Can you work these out from the drawing? Everything is in mm from the part's minimum corner. A direction names the side the tool comes from. Give positions to 0.01 mm unless a question says otherwise; leave off trailing zeros.
Q1. We'd pull the mould along X, two halves only. Please class the marked faces 3, 4 and 5: +X half, -X half, draft (parallel to the pull), parting line (faces both ways), or undercut.
Q2. For the marked faces 1 and 2, which set-ups out of +Z, -Z, +X, -X, +Y, -Y let a thin tool reach every point of the face, with its end or its side?
Q3. If we section it at A-A (y = 5): Give the number of separate pieces and of enclosed holes in the cut face.
Q4. I need wall thicknesses on line 1 (Z direction, x = 1.5, y = 5.75); line 2 (X direction, y = 6.25, z = 1.65); line 3 (Y direction, x = 14.75, z = 1.7) (1 decimal). Which ranges of each line are inside material? Lowest first, please.
Q5. Will these pins go through, and if not, where does the flat tip stop? P1, Ø2, axis at x = 12, z = 1, coming from the +Y side (1 decimal); P2, Ø1.5, axis at x = 6.5, z = 1, coming from the -Y side (1 decimal).
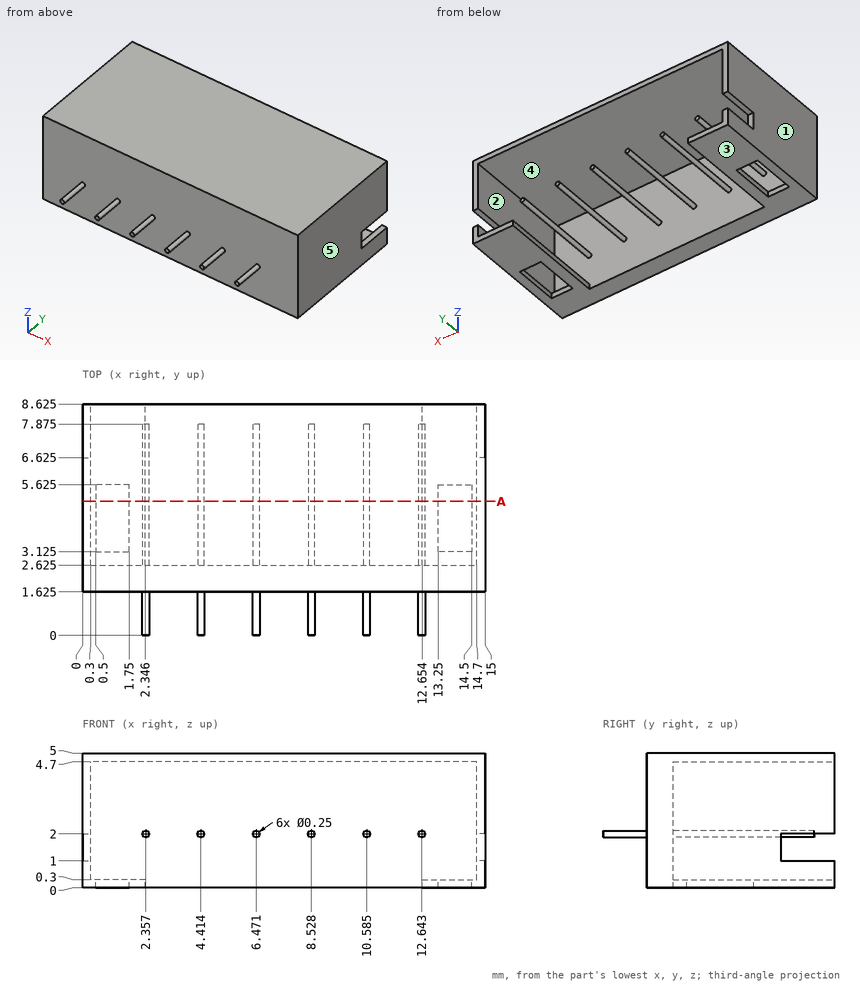
Check sheet entries:
1. face 3: draft
1. face 4: undercut
1. face 5: +X half
2. face 1: +Z, -Z, -X, +Y, -Y
2. face 2: +Y
3. separate pieces: 9
3. enclosed holes: 0
4. line 1: z = 0 to 0.3, 4.7 to 5
4. line 2: x = 0 to 0.3, 14.7 to 15
4. line 3: y = 1.6 to 6.6
5. P1: stops at y = 8.6
5. P2: stops at y = 1.6
